Autodesk Inventor part; units mm, degrees
ref_plane "YZ Plane" through (0, 0, 0) normal (1, 0, 0) x (0, 1, 0)
ref_plane "XZ Plane" through (0, 0, 0) normal (0, 1, 0) x (-1, 0, 0)
ref_plane "XY Plane" through (0, 0, 0) normal (0, 0, 1) x (1, 0, 0)
sketch "Эскиз2" plane through (0, 0, 0) normal (0, 0, 1) x (1, 0, 0)
  line L0 (0, 0) -> (25, 0)
  line L1 (0, 0) -> (0, 15)
  line L2 (0, 15) -> (25, 0)
  line L3 (0, -3) -> (0, 18)
  dimension "d0" = 25
  dimension "d1" = 15
revolve "Вращение1" add sketch "Эскиз2" angle 360 about axis through (0, -10, 0) along (0, 1, 0)
ref_plane "РабПлоскость1" through (0, 10, 0) normal (0, -1, 0) x (1, 0, 0)
sketch "Эскиз3" plane through (0, 10, 0) normal (0, -1, 0) x (1, 0, 0)
  line L0 (9.9198, 18.1472) -> (-9.6073, 18.1472)
  line L1 (-9.6073, 18.1472) -> (-9.6073, -14.8146)
  line L2 (-9.6073, -14.8146) -> (9.9198, -14.8146)
  line L3 (9.9198, -14.8146) -> (9.9198, 18.1472)
  point P0 (0, 0)
extrude "Выдавливание1" cut sketch "Эскиз3" against normal blind 10
sketch "Эскиз4" plane through (0, 0, 0) normal (1, 0, 0) x (0, 1, 0)
  line L0 (14.521, 7.5) -> (0, 7.5)
  line L1 (0, 7.5) -> (0, -7.5)
  line L2 (0, -7.5) -> (14.521, -7.5)
  line L3 (14.521, -7.5) -> (14.521, 7.5)
  line L4 (14.521, 7.5) -> (0, -7.5) construction
  line L5 (0, 7.5) -> (14.521, -7.5) construction
  line L6 (10, 8.3333) -> (10, -8.3333)
  arc A0 (7.0249, 0.2433) -> (7.0249, -0.2433) centre (14.521, 0) ccw
  arc A1 (14.521, -7.5) -> (14.521, 7.5) centre (14.521, 0) ccw
  line L7 (14.521, 0) -> (17.021, 0) construction
  circle A2 centre (17.021, 0) radius 1.55
  point P0 (0, 0)
  point P1 (7.2605, 0)
  point P2 (10, 7.5)
  point P3 (10, -7.5)
  dimension "d6" = 15
  dimension "d7" = 4.521
  dimension "d10" = 2.5
  dimension "d11" = 3.1
extrude "Выдавливание2" add sketch "Эскиз4" along normal mid plane 20 contours L3 L2 L6 L0 | A1 L3
extrude "Выдавливание3" cut sketch "Эскиз4" along normal mid plane 10 contours A1 L3 | L6 L2 L1 L0
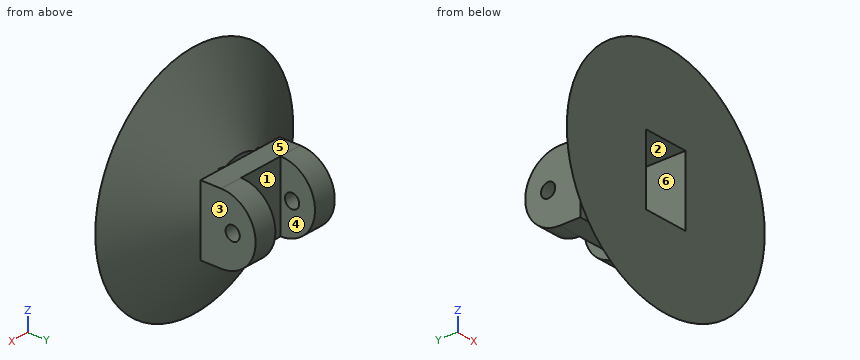
Verification items for the finished model (mm, model axes). Face numbers are marked on the shaded views. A direction names the side the tool comes from. Give positions to 0.01 mm unless a question says otherwise; leave off trailing zeros. Order: outer loops, then holes, each group sorted by start corner. A loop starts at its lowest first (then second) coordinate and runs counter-clockwise, first axis right, second up. Notation, with made-up numbers: (82.5, 34) - (111.5, 34) arc R14 ccw to (111.5, 55) - close; hole circle Ø3 at (70.25, 87.25). An arc over 180 degrees is marked (long way). Answer as CSV lines item,"result". Start each with the question number.
Item 1: Access from +Z, -Z, +X, -X, +Y, -Y to the whole of each face (thin tool, end or side, straight path). Record for the marked faces 1, 2 and 3.
Item 2: Section check C-C, the plane y = 17.75. Record the boundary of the cut face in (x, z).
Item 3: Section check A-A, the plane z = 0. Record the boundary of the cut face in (x, y), plus the area to 3 significant figures.
Item 4: Material ranges on L1, parallel to Y at x = -9, z = -0.5; L2, parallel to Z at x = -4, y = 10.75; L3, parallel to Y at x = 0, z = 5, recorded low to high.
Item 5: Mould release check, pull along Z, two halves, no side actions. Record for the marked faces 4, 5 and 6: released by +Z, released by -Z, zero draft, split by the parting line, or undercut.
Item 6: Section check D-D, the plane y = 20.5. Record the boundary of the cut face in (x, z), plus the area to 3 significant figures.
Item 7: Gauge pin test, flat ends, axial feed: pin 1 (11 mm diameter, centred on x = 1.5, y = 3, fed in from -Z); pin 2 (9.5 mm diameter, centred on y = 14, z = -0.5, fed in from +X); pin 3 (1 mm diameter, centred on x = -1.5, y = 12, fed in from -Z). Record the tip position at first contact, or that the pin passes through.
Filled in:
1,face 1,"+Z, -Z, +Y"
1,face 2,"-Y"
1,face 3,"+Z, -Z, +X, +Y"
2,outline,"(-10, -6.77) - (-5, -6.77) - (-5, -1.37) - (-10, -1.37) - close; (-10, 1.37) - (-5, 1.37) - (-5, 6.77) - (-10, 6.77) - close; (5, -6.77) - (10, -6.77) - (10, -1.37) - (5, -1.37) - close; (5, 1.37) - (10, 1.37) - (10, 6.77) - (5, 6.77) - close"
3,outline,"(-25, 0) - (-5, 0) - (-5, 10) - (5, 10) - (5, 0) - (25, 0) - (8.33, 10) - (10, 10) - (10, 15.47) - (5, 15.47) - (5, 14.52) - (-5, 14.52) - (-5, 15.47) - (-10, 15.47) - (-10, 10) - (-8.33, 10) - close; (-10, 18.57) - (-5, 18.57) - (-5, 22.02) - (-10, 22.02) - close; (5, 18.57) - (10, 18.57) - (10, 22.02) - (5, 22.02) - close"
3,area,"368 mm^2"
4,L1,"0 to 9.59, 10 to 15.55, 18.49 to 22"
4,L2,"-7.5 to 7.5"
4,L3,"10 to 14.52"
5,face 4,"zero draft"
5,face 5,"released by +Z"
5,face 6,"undercut"
6,outline,"(-10, -4.53) - (-5, -4.53) - (-5, 4.53) - (-10, 4.53) - close; (5, -4.53) - (10, -4.53) - (10, 4.53) - (5, 4.53) - close"
6,area,"90.6 mm^2"
7,pin 1,"z = -25"
7,pin 2,"x = 10"
7,pin 3,"z = -7.5"
